```python
from build123d import *

# Parameters (mm, degrees)
F0_W      = 101.6
F0_H      = 101.6
F1_DEPTH  = 12.7
F2_W      = 12.7
F2_H      = 12.7
F3_DEPTH  = 12.701
F4_W      = 12.7
F4_H      = 12.7
F5_DEPTH  = 12.701
F6_W      = 6.35
F6_H      = 5.423685
F7_DEPTH  = 88.901
F8_W      = 6.35
F8_H      = 5.389227
F9_DEPTH  = 88.901
F10_R     = 9.525
F11_DEPTH = 12.701


with BuildPart() as f1:
    # F0 (on Top) → F1 (new body)
    with BuildSketch(Plane.XY):
        Rectangle(F0_W, F0_H)
    extrude(amount=F1_DEPTH)

    # F2 (on face) → F3 (cut, through all)
    with BuildSketch(Plane.XY.offset(12.7)):
        with Locations((-44.45, 19.05)):
            Rectangle(F2_W, F2_H)
        with Locations((-44.45, 44.45)):
            Rectangle(F2_W, F2_H)
        with Locations((-44.45, -6.35)):
            Rectangle(F2_W, F2_H)
        with Locations((-44.45, -31.75)):
            Rectangle(F2_W, F2_H)
    extrude(amount=-F3_DEPTH, mode=Mode.SUBTRACT)

    # F4 (on face) → F5 (cut, through all)
    with BuildSketch(Plane.XY.offset(12.7)):
        with Locations((44.45, 31.75)):
            Rectangle(F4_W, F4_H)
        with Locations((44.45, 6.35)):
            Rectangle(F4_W, F4_H)
        with Locations((44.45, -19.05)):
            Rectangle(F4_W, F4_H)
        with Locations((44.45, -44.45)):
            Rectangle(F4_W, F4_H)
    extrude(amount=-F5_DEPTH, mode=Mode.SUBTRACT)

    # F6 (on face) → F7 (cut, through all)
    with BuildSketch(Plane.YZ.offset(38.1)):
        with Locations((-41.275, 2.711842)):
            Rectangle(F6_W, F6_H)
    extrude(amount=-F7_DEPTH, mode=Mode.SUBTRACT)

    # F8 (on face) → F9 (cut, through all)
    with BuildSketch(Plane(origin=(-38.1, 0, 0), x_dir=(0, -1, 0), z_dir=(-1, 0, 0))):
        with Locations((-41.275, 2.694613)):
            Rectangle(F8_W, F8_H)
    extrude(amount=-F9_DEPTH, mode=Mode.SUBTRACT)

    # F10 (on face) → F11 (cut, through all)
    with BuildSketch(Plane.XY.offset(12.7)):
        Circle(F10_R)
    extrude(amount=-F11_DEPTH, mode=Mode.SUBTRACT)


solid = f1.part
```
Work out the finished part from the listing and answer in its coordinate system (mm). A direction names the side the tool comes from. Coordinates: 2 decimals unless noted, no trailing zeros. Write each loop counter-clockwise with the first axis right and the second up, starting at its lowest first coordinate (ties: lowest second). Pieces come first, ordered by that corner, then holes. Notation, with made-up numbers: (57, -39.5) - (106, -39.5) arc R19 ccw to (106, -25.5) - close; hole circle Ø11 at (10, 64). An arc over 180 degrees is marked (long way). Answer as a JSON object with one key per item and string values.
Q1. Find section D-D (x = 19.5). Write down the section's boundary in (y, z).
Results list:
{"outline": "(-50.8, 0) - (-44.45, 0) - (-44.45, 5.42) - (-38.1, 5.42) - (-38.1, 0) - (38.1, 0) - (38.1, 5.39) - (44.45, 5.39) - (44.45, 0) - (50.8, 0) - (50.8, 12.7) - (-50.8, 12.7) - close"}
Q2. Find section B-B (x = 0). Write down the section's boundary in (y, z) (3 decimals), plus the area to 3 significant figures.
Results list:
{"outline": "(-50.8, 0) - (-44.45, 0) - (-44.45, 5.424) - (-38.1, 5.424) - (-38.1, 0) - (-9.525, 0) - (-9.525, 12.7) - (-50.8, 12.7) - close; (9.525, 0) - (38.1, 0) - (38.1, 5.389) - (44.45, 5.389) - (44.45, 0) - (50.8, 0) - (50.8, 12.7) - (9.525, 12.7) - close", "area": "980 mm^2"}
Q3. Find section A-A (z = 1.25). State how many separate pieces and enclosed holes the cut face has, plus the area to 3 significant figures.
Results list:
{"separate pieces": "3", "enclosed holes": "1", "area": "7,620 mm^2"}
Q4. Given pin 1 Ø6.5 at (y, z) = (-7, 5.5) entering from -X; pin 2 Ø6.5 at (y, z) = (6.5, 8.5) entering from +X; pin 3 Ø6 at (x, z) = (-44, 9) entering from +Y, each flat-ended and moving along its own axis, determine where each tip first touches the part or whether it passes through.
Results list:
{"pin 1": "stops at x = -38.1", "pin 2": "stops at x = 38.1", "pin 3": "stops at y = 38.1"}
Q5. Consider L1, parallel to Y at x = -28.5, z = 2.5; L2, parallel to Y at x = 0, z = 4.25 (3 decimals); L3, parallel to Y at x = 0, z = 6.25 (3 decimals). Determine where each line is inside the solid, lowest interval first. Write a range as from..to.
Results list:
{"L1": "y = -50.8..-44.45, -38.1..38.1, 44.45..50.8", "L2": "y = -50.8..-44.45, -38.1..-9.525, 9.525..38.1, 44.45..50.8", "L3": "y = -50.8..-9.525, 9.525..50.8"}
Q6. Which of the six approach directions +Z, -Z, +X, -X, +Y, -Y give full straight-line access (tool end or side, diameter ignored) to faces 1 (the flat face through (7, -38.1, 3)), 2 (the flat face through (-45, -38.1, 9)), 3 (the flat face through (-6, -41, 5.424)), 4 (the flat face through (38.1, -46, 8))?
Results list:
{"face 1": "-Z, +X", "face 2": "+Z, -Z, -X", "face 3": "-Z, +X, -X", "face 4": "+Z, -Z, +X, -Y"}
Q7. For a pull along Y with two mould halves and no side action, classify faces 5 (the flat face through (-45, 12.7, 6)), 6 (the flat face through (-7, -48, 0)) as pulls with the +Y half, pulls with the -Y half, needs draft (parallel to the pull), parting line crosses it, or undercut.
Results list:
{"face 5": "undercut", "face 6": "needs draft"}
